```python
from build123d import *

# Parameters (mm, degrees)
SALIENTE_EXTRUIR1_DEPTH = 2
CROQUIS9_R              = 1.5
CORTAR_EXTRUIR5_DEPTH   = 6


with BuildPart() as part:
    # Croquis1 → Saliente-Extruir1 (new body)
    with BuildSketch(Plane.XY):
        Polygon((0, 0), (60, 0), (60, 80), (-24, 80), (-24, 20.138391148), align=None)
    extrude(amount=SALIENTE_EXTRUIR1_DEPTH)

    # Croquis9 → Cortar-Extruir5 (cut)
    with BuildSketch(Plane.XY.offset(2)):
        with Locations((-21.807968978, 77.807968978)):
            Circle(CROQUIS9_R)
        with Locations((-21.91549209, 21.11041315)):
            Circle(CROQUIS9_R)
        with Locations((0.764337492, 2.1)):
            Circle(CROQUIS9_R)
        with Locations((55, 78)):
            Circle(CROQUIS9_R)
        with Locations((55, 2)):
            Circle(CROQUIS9_R)
    extrude(amount=-CORTAR_EXTRUIR5_DEPTH, mode=Mode.SUBTRACT)


solid = part.part
```
Geometry: final body of the model. Coordinates: model frame, mm. Round coordinates to 2 decimals unless told otherwise and drop trailing zeros. Order: outer loops, then holes, each group sorted by start corner. A loop starts at its lowest first (then second) coordinate and runs counter-clockwise, first axis right, second up. Notation, with made-up numbers: (70.25, 5) -> (87.25, 5) arc R26 ccw to (87.25, 26) -> close; hole circle Ø10 at (-30.5, 78.5). An arc over 180 degrees is marked (long way). Use CSV: the item, a comma, the result in double quotes. Start each with the question number.
1) Section C-C (y = 9.5). Return the cut outline in (x, z), and give its area (3 significant figures).
2) Section A-A (x = 55). Return the cut outline in (y, z).
3) Draft query along X for faces 1 (the face through (60, 39, 1)), 2 (the face through (30, 0, 1)), 3 (the face through (55.806, 79.265, 1.014)), 4 (the face through (-22.003, 79.295, 1.014)). Return one class per face: +X half, -X half, draft (parallel to the pull), parting line (faces both ways), or undercut.
4) Material intervals for line 1 along Y through (x, z) = (55, 1); line 2 along X through (y, z) = (78, 1.4); line 3 along X through (y, z) = (20, 1.75), sorted ascending. Write a range as from..to.
5) Section D-D (x = -12). Return the cut outline in (y, z).
6) Section B-B (z = 0.6). Return the cut outline in (x, y).
7) First-contact query: pin 1 Ø5 at (x, y) = (55, 2) entering from +Z. Flat tip, straight axial feed; report the tip coordinate or a pass-through.
Returned:
1,outline,"(-11.32, 0) -> (60, 0) -> (60, 2) -> (-11.32, 2) -> close"
1,area,"143 mm²"
2,outline,"(0, 0) -> (0.5, 0) -> (0.5, 2) -> (0, 2) -> close; (3.5, 0) -> (76.5, 0) -> (76.5, 2) -> (3.5, 2) -> close; (79.5, 0) -> (80, 0) -> (80, 2) -> (79.5, 2) -> close"
3,face 1,"+X half"
3,face 2,"draft"
3,face 3,"undercut"
3,face 4,"undercut"
4,line 1,"y = 0..0.5, 3.5..76.5, 79.5..80"
4,line 2,"x = -24..-23.3, -20.32..53.5, 56.5..60"
4,line 3,"x = -23.84..-22.92, -20.91..60"
5,outline,"(10.07, 0) -> (80, 0) -> (80, 2) -> (10.07, 2) -> close"
6,outline,"(-24, 20.14) -> (0, 0) -> (60, 0) -> (60, 80) -> (-24, 80) -> close; hole circle Ø3 at (-21.92, 21.11); hole circle Ø3 at (-21.81, 77.81); hole circle Ø3 at (0.76, 2.1); hole circle Ø3 at (55, 2); hole circle Ø3 at (55, 78)"
7,pin 1,"stops at z = 2"
